from build123d import *

# Parameters (mm, degrees)
F0_R     = 1.524
F1_DEPTH = 6.35
F2_R     = 1.2573
F3_DEPTH = 25.4
F4_R     = 0.635


with BuildPart() as f1:
    # F0 (on Top) → F1 (new body)
    with BuildSketch(Plane.XY):
        with Locations((-16.261026, 27.197644)):
            Circle(F0_R)
    extrude(amount=F1_DEPTH)

    # F2 (on face) → F3 (join)
    with BuildSketch(Plane(origin=(0, 0, 0), x_dir=(1, 0, 0), z_dir=(0, 0, -1))):
        with Locations((-16.261026, -27.197644)):
            Circle(F2_R)
    extrude(amount=F3_DEPTH)

    # F4
    f4_edges = [f1.edges().sort_by_distance(p)[0] for p in [
        (-17.518326, 27.197644, -25.4),
    ]]
    fillet(f4_edges, radius=F4_R)


solid = f1.part
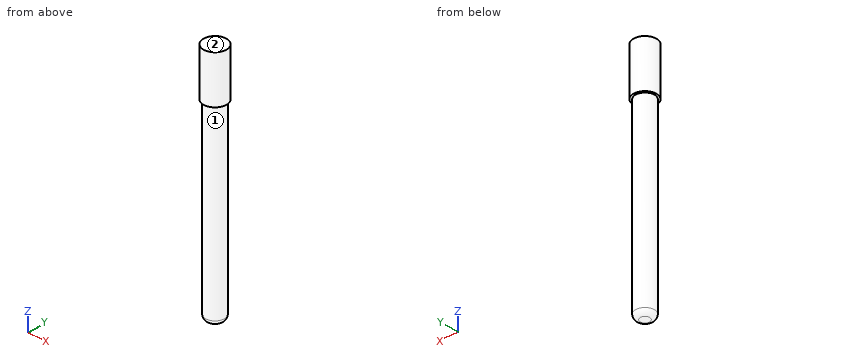
Verification items for the finished model (mm, model axes). Face numbers are marked on the shaded views. A direction names the side the tool comes from. Give positions to 0.01 mm unless a question says otherwise; leave off trailing zeros. Write each loop counter-clockwise with the first axis right and the second up, starting at its lowest first coordinate (ties: lowest second). Pieces come first, ordered by that corner, then holes. Notation, with made-up numbers: (-34, 47) - (16, 47) arc R20 cw to (16, 63) - close; hole circle Ø8 at (-14, 34.25). An arc over 180 degrees is marked (long way). Answer as CSV lines item,"result". Start each with the question number.
1. Sectioned sample at A-A (z = -2.5). Record the boundary of the cut face in (x, y), then the cut area to 3 significant figures.
2. Thickness scan on line 1 (Z direction, x = -16, y = 28.55); line 2 (Y direction, x = -16.3, z = -11); line 3 (X direction, y = 26.45, z = -8.5). Record the ranges inside material, lowest first.
3. Set-up check for the marked faces 1 and 2: record each of +Z, -Z, +X, -X, +Y, -Y from which the full face is reachable in a straight line by a thin tool's end or side.
4. Depth check by flat-ended pin: pin 1 (1.5 mm diameter, centred on x = -15.5, z = -18.5, fed in from -Y); pin 2 (1.5 mm diameter, centred on y = 26, z = 2, fed in from -X). Enter the tip coordinate at first touch or a pass-through.
Derived:
1,outline,"circle Ø2.51 at (-16.26, 27.2)"
1,area,"4.97 mm²"
2,line 1,"0 to 6.35"
2,line 2,"25.94 to 28.45"
2,line 3,"-17.27 to -15.25"
3,face 1,"-Z"
3,face 2,"+Z, +X, -X, +Y, -Y"
4,pin 1,"y = 25.94"
4,pin 2,"x = -17.72"
